Design review of the part shown in the three views and the two pictorial views. Dimensions are in mm from the part's minimum x, y and z. A direction names the side the tool comes from. Round coordinates to 2 decimals unless told otherwise and drop trailing zeros. Loops run counter-clockwise (first coordinate to the right, second up) from the corner with the lowest first, then second, coordinate; pieces in that order, holes last. Notation, with made-up numbers: (29.25, -31) -> (33.25, -31) arc R22 ccw to (33.25, 7) -> close; hole circle Ø2 at (72.5, 4.5). An arc over 180 degrees is marked (long way). Use a Markdown table: item, result. Add a question column.
1) Consider section B-B on y = 27. Give the boundary of the cut face in (x, z), plus the area to 3 significant figures.
2) Consider section C-C on z = 96. Give the boundary of the cut face in (x, y), plus the area to 3 significant figures.
3) For the marked faces 1, 2 and 3, list the 3-axis set-ups (+Z, -Z, +X, -X, +Y, -Y) from which the entire face can be reached by the end or side of a thin tool; tool diameter is ignored.
4) Consider section A-A on x = 88. Give the boundary of the cut face in (y, z).
5) Wall thickness on probe 1 along Z at (x, y) = (9, 5); probe 2 along X at (y, z) = (18, 91.5); probe 3 along Y at (x, z) = (23.5, 111): over which ranges is each line inside the solid? List them lowest first.
6) Consider section D-D on x = 14. Give the boundary of the cut face in (y, z).
7) Insertion check: pin 1 (4 mm diameter, centred on y = 31, z = 107, fed in from +X); pin 2 (8 mm diameter, centred on y = 10, z = 56.5, fed in from +X); pin 3 (10 mm diameter, centred on x = 80, y = 29, fed in from -Z). Each pin has a flat end and moves straight along its axis. Give the tip position at first contact, or say it passes through.
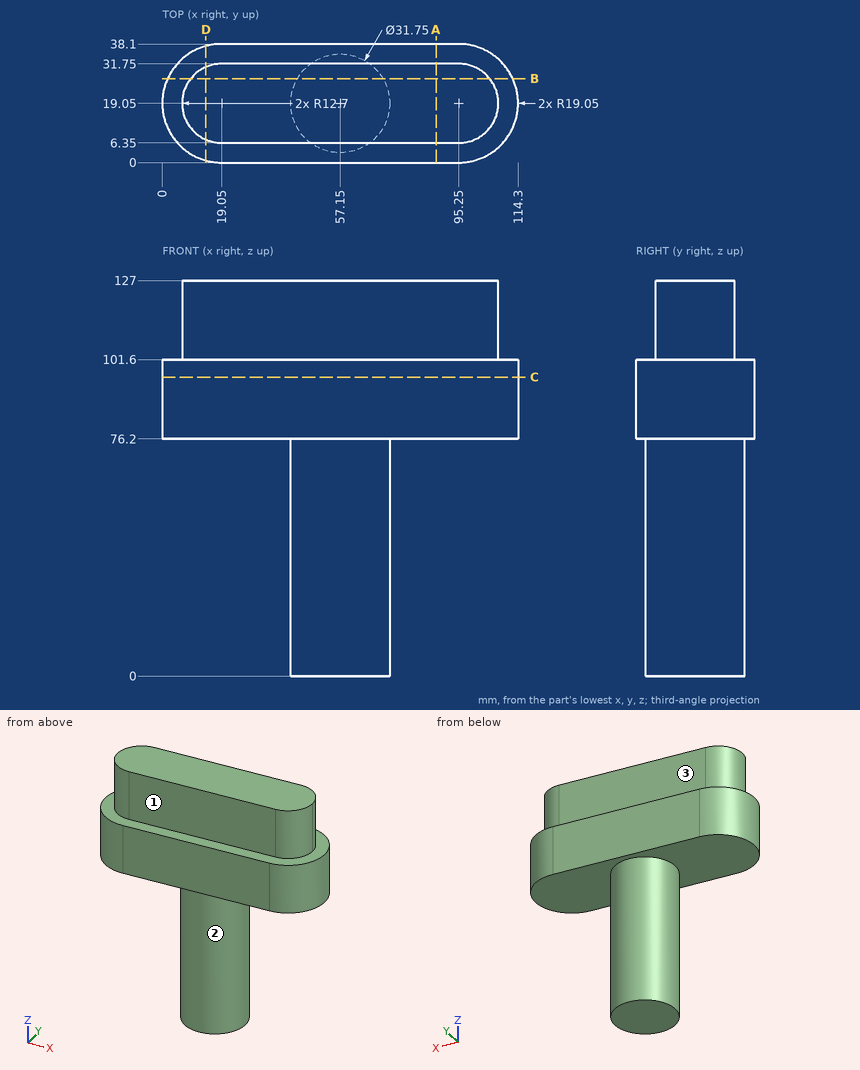
Result set:
| question | item | result |
|---|---|---|
| 1 | outline | (1.74, 76.2) -> (43.41, 76.2) -> (43.41, 0) -> (70.89, 0) -> (70.89, 76.2) -> (112.56, 76.2) -> (112.56, 101.6) -> (105.15, 101.6) -> (105.15, 127) -> (9.15, 127) -> (9.15, 101.6) -> (1.74, 101.6) -> close |
| 1 | area | 7,350 mm2 |
| 2 | outline | (19.05, 0) -> (95.25, 0) arc R19.05 ccw to (95.25, 38.1) -> (19.05, 38.1) arc R19.05 ccw to start |
| 2 | area | 4,040 mm2 |
| 3 | face 1 | +Z, +X, -X, -Y |
| 3 | face 2 | -Z |
| 3 | face 3 | +Z, +X, -X, +Y |
| 4 | outline | (0, 76.2) -> (38.1, 76.2) -> (38.1, 101.6) -> (31.75, 101.6) -> (31.75, 127) -> (6.35, 127) -> (6.35, 101.6) -> (0, 101.6) -> close |
| 5 | probe 1 | 76.2 to 101.6 |
| 5 | probe 2 | 0.03 to 114.27 |
| 5 | probe 3 | 6.35 to 31.75 |
| 6 | outline | (0.68, 76.2) -> (37.42, 76.2) -> (37.42, 101.6) -> (30.7, 101.6) -> (30.7, 127) -> (7.4, 127) -> (7.4, 101.6) -> (0.68, 101.6) -> close |
| 7 | pin 1 | x = 103.14 |
| 7 | pin 2 | x = 72.2 |
| 7 | pin 3 | z = 76.2 |
